Input: dimensioned drawing with shaded views. Units: mm. Origin: part minimum x, y, z. A direction names the side the tool comes from. Give positions to 0.01 mm unless a question says otherwise; leave off trailing zeros. Order: outer loops, then holes, each group sorted by start corner. A loop starts at its lowest first (then second) coordinate and runs counter-clockwise, first axis right, second up.
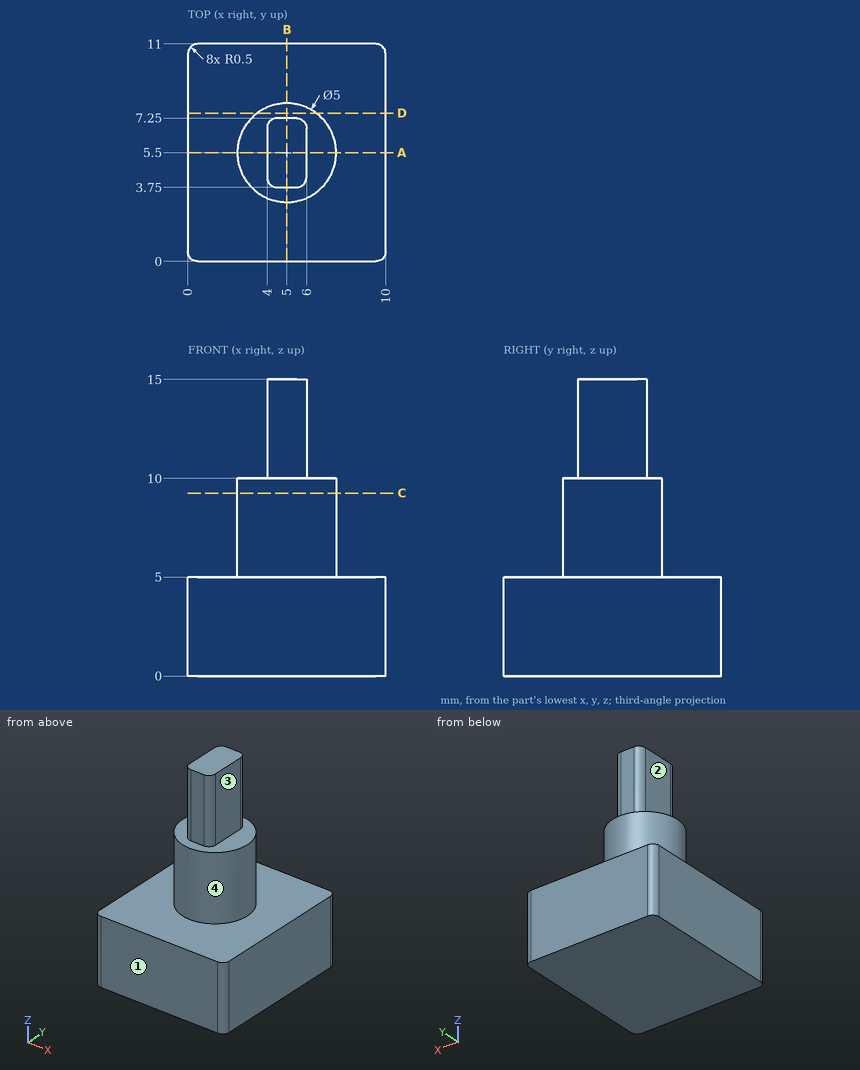
1) Material intervals for L1, parallel to Z at x = 6, y = 9.5; L2, parallel to Z at x = 7, y = 6.5; L3, parallel to X at y = 6.5, z = 8.5, sorted ascending.
Report:
L1: z = 0 to 5
L2: z = 0 to 10
L3: x = 2.71 to 7.29
2) Pin query (flat end, axial travel): pin 1 (0.8 mm diameter, centred on y = 6, z = 12, fed in from -X); pin 2 (6 mm diameter, centred on y = 5, z = 8.5, fed in from -X); pin 3 (3 mm diameter, centred on y = 6, z = 12.5, fed in from +X). Return the tip coordinate at first contact, or that it passes through.
Report:
pin 1: stops at x = 4
pin 2: stops at x = 2.5
pin 3: stops at x = 6
3) Section query C-C, the plane z = 9.25. Return the cut outline in (x, y).
Report:
outline: circle Ø5 at (5, 5.5)
4) Section query A-A, the plane y = 5.5. Return the cut outline in (x, z), and give its area (3 significant figures).
Report:
outline: (0, 0) - (10, 0) - (10, 5) - (7.5, 5) - (7.5, 10) - (6, 10) - (6, 15) - (4, 15) - (4, 10) - (2.5, 10) - (2.5, 5) - (0, 5) - close
area: 85.0 mm2
5) Section query B-B, the plane x = 5. Return the cut outline in (y, z), and give its area (3 significant figures).
Report:
outline: (0, 0) - (11, 0) - (11, 5) - (8, 5) - (8, 10) - (7.25, 10) - (7.25, 15) - (3.75, 15) - (3.75, 10) - (3, 10) - (3, 5) - (0, 5) - close
area: 97.5 mm2
6) Section query D-D, the plane y = 7.5. Return the cut outline in (x, z).
Report:
outline: (0, 0) - (10, 0) - (10, 5) - (6.5, 5) - (6.5, 10) - (3.5, 10) - (3.5, 5) - (0, 5) - close
7) Reachability of the marked faces 1, 2, 3 and 4 from +Z, -Z, +X, -X, +Y, -Y: full face, straight path, thin tool, end or side. Return the list, or none.
Report:
face 1: +Z, -Z, +X, -X, -Y
face 2: +Z, -X, +Y, -Y
face 3: +Z, +X, +Y, -Y
face 4: +Z
